Autodesk Inventor part; units mm, degrees
ref_plane "YZ Plane" through (0, 0, 0) normal (1, 0, 0) x (0, 1, 0)
ref_plane "XZ Plane" through (0, 0, 0) normal (0, 1, 0) x (-1, 0, 0)
ref_plane "XY Plane" through (0, 0, 0) normal (0, 0, 1) x (1, 0, 0)
sketch "Sketch1" plane through (0, 0, 0) normal (0, 0, 1) x (1, 0, 0)
  line L0 (-4.8, 0) -> (0.8, 0) construction
  line L1 (0, -37.1) -> (0, 37.1) construction
  line L2 (-4, 26.5) -> (0, 26.5)
  line L3 (0, 26.5) -> (0, -26.5)
  line L4 (0, -26.5) -> (-4, -26.5)
  line L5 (-4, -26.5) -> (-4, 26.5)
  point P0 (0, 0)
  dimension "d1" = 53
  dimension "d16" = 8
revolve "Revolution1" add sketch "Sketch1" angle 360 about axis through (0, -10, 0) along (0, 1, 0)
sketch "Sketch2" plane through (0, 26.5, 0) normal (0, 1, 0) x (1, 0, 0)
  circle A0 centre (0, 0) radius 4
hole "Hole1" at (0, 26.5, 0) direction (0, -1, 0) diameter 2.459 depth 15 tip angle 118
mirror "Espelhar1" [suppressed]
chamfer "Chamfer1" distance 0.5 angle 45 2 edges at (4, -26.5, 0) (4, 26.5, 0)
chamfer "Chamfer2" distance 0.3 angle 45 1 edges at (0, 26.5, -1.2295)
properties part number "GRJ-05-104" material "Poliacetal WT"
Design review of the part built by this model. Coordinates are the model's own, in mm. Round coordinates to 2 decimals unless told otherwise and drop trailing zeros. Write each loop counter-clockwise with the first axis right and the second up, starting at its lowest first coordinate (ties: lowest second). Pieces come first, ordered by that corner, then holes.
Item 1: Consider section A-A on y = -16.5. Give the boundary of the cut face in (x, z).
Item 2: For pin 1 Ø1.5 at (y, z) = (6.5, -2) entering from +X; pin 2 Ø1.5 at (y, z) = (3.5, -1) entering from -X, all flat-tipped, find the tip position at first contact; note any pin that passes through.
Item 3: Wall thickness on L1, parallel to Z at x = 0, y = 19.25; L2, parallel to Z at x = -3, y = -14.5; L3, parallel to X at y = 22, z = 1: over which ranges is each line inside the solid? List them lowest first.
Item 4: Draft analysis for pull direction Z (two halves, no side actions). For faces 1 (the conical face through (-0.21, 10.89, -0.05)), 2 (the cylindrical face through (0.867, 0.364, -3.905)), 3 (the cylindrical face through (0.748, 18.747, -0.976)), 4 (the flat face through (-1, 26.5, -2)), state which applies: released by +Z, released by -Z, zero draft, split by the parting line, or undercut.
Check values:
1. outline: circle Ø8 at (0, 0)
2. pin 1: stops at x = 3.8
2. pin 2: stops at x = -3.99
3. L1: z = -4 to -1.23, 1.23 to 4
3. L2: z = -2.65 to 2.65
3. L3: x = -3.87 to -0.72, 0.72 to 3.87
4. face 1: undercut
4. face 2: split by the parting line
4. face 3: undercut
4. face 4: zero draft
